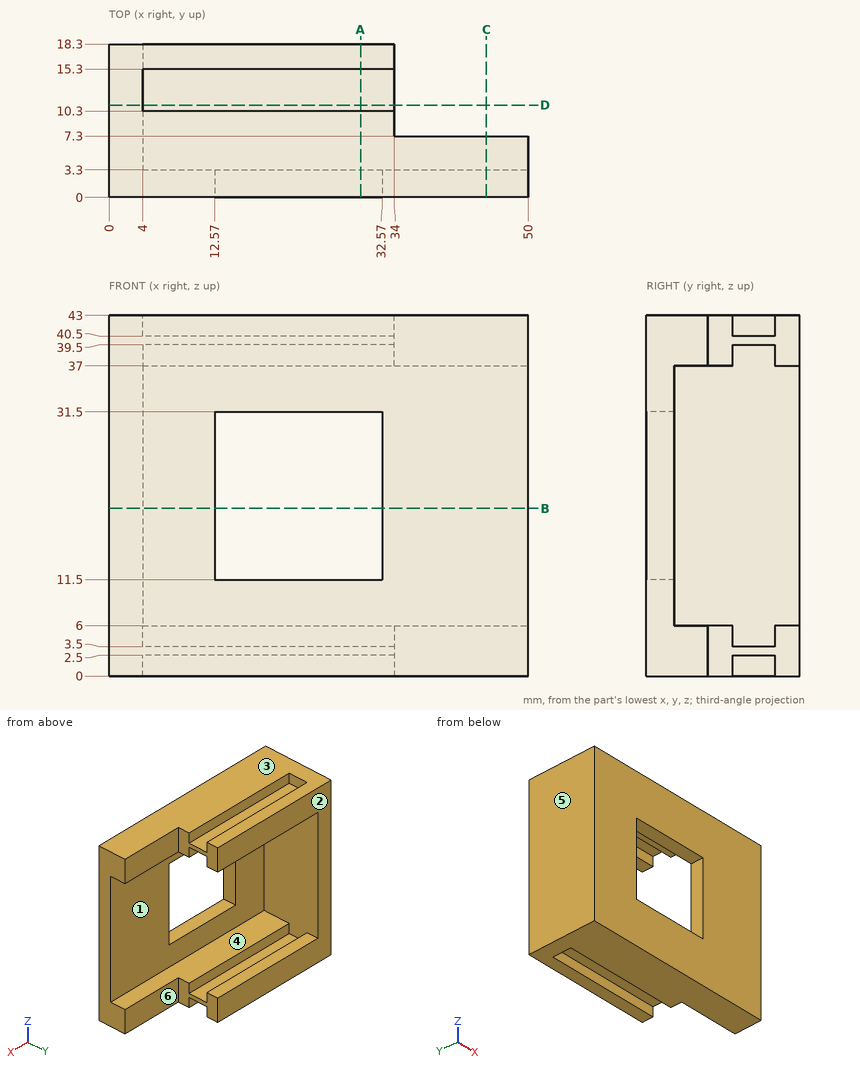
Verification items for this drawing (mm, ordinates from the low corner). A direction names the side the tool comes from. Coordinates: 2 decimals unless noted, no trailing zeros. Loops run counter-clockwise (first coordinate to the right, second up) from the corner with the lowest first, then second, coordinate; pieces in that order, holes last. Notation, with made-up numbers: (-19.5, -15) -> (38.5, -15) arc R22 ccw to (38.5, 8) -> close; hole circle Ø4 at (46, -39). An arc over 180 degrees is marked (long way). Put each result on its own line as item: value.
1. Section check D-D, the plane y = 11. Record the boundary of the cut face in (x, z).
Result set:
outline: (0, 0) -> (4, 0) -> (4, 2.5) -> (34, 2.5) -> (34, 3.5) -> (4, 3.5) -> (4, 39.5) -> (34, 39.5) -> (34, 40.5) -> (4, 40.5) -> (4, 43) -> (0, 43) -> close
2. Gauge pin test, flat ends, axial feed: P1, Ø3, axis at x = 43.5, z = 40.5, coming from the +Y side; P2, Ø5, axis at y = 11.5, z = 40.5, coming from the +X side; P3, Ø15.5, axis at x = 18.5, z = 23, coming from the +Y side. Record the tip position at first contact, or that the pin passes through.
Result set:
P1: stops at y = 7.3
P2: stops at x = 34
P3: stops at y = 3.3
3. Section check B-B, the plane z = 20. Record the boundary of the cut face in (x, y).
Result set:
outline: (0, 0) -> (12.57, 0) -> (12.57, 3.3) -> (4, 3.3) -> (4, 18.3) -> (0, 18.3) -> close; (32.57, 0) -> (50, 0) -> (50, 3.3) -> (32.57, 3.3) -> close
4. Mould release check, pull along Z, two halves, no side actions. Record for the marked faces 1, 2 and 3: pulls with the +Z half, pulls with the -Z half, needs draft (parallel to the pull), parting line crosses it, or undercut.
Result set:
face 1: undercut
face 2: needs draft
face 3: pulls with the +Z half
5. Tool access check on the marked faces 4, 5 and 6. Record the directions out of +Z, -Z, +X, -X, +Y, -Y that give a thin tool (end or side, any length) a straight path to the whole face; none if there is none.
Result set:
face 4: +X, +Y
face 5: +Z, -Z, -X, +Y, -Y
face 6: +Z, -Z, +X, +Y
6. Section check A-A, the plane x = 30. Record the boundary of the cut face in (y, z).
Result set:
outline: (0, 0) -> (10.3, 0) -> (10.3, 2.5) -> (15.3, 2.5) -> (15.3, 0) -> (18.3, 0) -> (18.3, 6) -> (15.3, 6) -> (15.3, 3.5) -> (10.3, 3.5) -> (10.3, 6) -> (3.3, 6) -> (3.3, 11.5) -> (0, 11.5) -> close; (0, 31.5) -> (3.3, 31.5) -> (3.3, 37) -> (10.3, 37) -> (10.3, 39.5) -> (15.3, 39.5) -> (15.3, 37) -> (18.3, 37) -> (18.3, 43) -> (15.3, 43) -> (15.3, 40.5) -> (10.3, 40.5) -> (10.3, 43) -> (0, 43) -> close
7. Thickness scan on line 1 (Z direction, x = 23, y = 3.75); line 2 (X direction, y = 1, z = 22); line 3 (Z direction, x = 33.5, y = 12). Record the ranges inside material, lowest first.
Result set:
line 1: z = 0 to 6, 37 to 43
line 2: x = 0 to 12.57, 32.57 to 50
line 3: z = 2.5 to 3.5, 39.5 to 40.5
8. Section check C-C, the plane x = 45. Record the boundary of the cut face in (y, z), then the cut area to 3 significant figures.
Result set:
outline: (0, 0) -> (7.3, 0) -> (7.3, 6) -> (3.3, 6) -> (3.3, 37) -> (7.3, 37) -> (7.3, 43) -> (0, 43) -> close
area: 190 mm^2
